The figure shows three views and two pictorial views of one solid part (mm, origin at its lowest corner). Answer the questions. A direction names the side the tool comes from. Coordinates: 2 decimals unless noted, no trailing zeros. Write each loop counter-clockwise with the first axis right and the second up, starting at its lowest first coordinate (ties: lowest second). Pieces come first, ordered by that corner, then holes. Notation, with made-up numbers: M 61,69.25 L 89,69.25 A28 cw 89,98.25 Z; hole C 70,26 d11. An arc over 180 degrees is marked long. Write item = value, one per line. Start each with the question number.
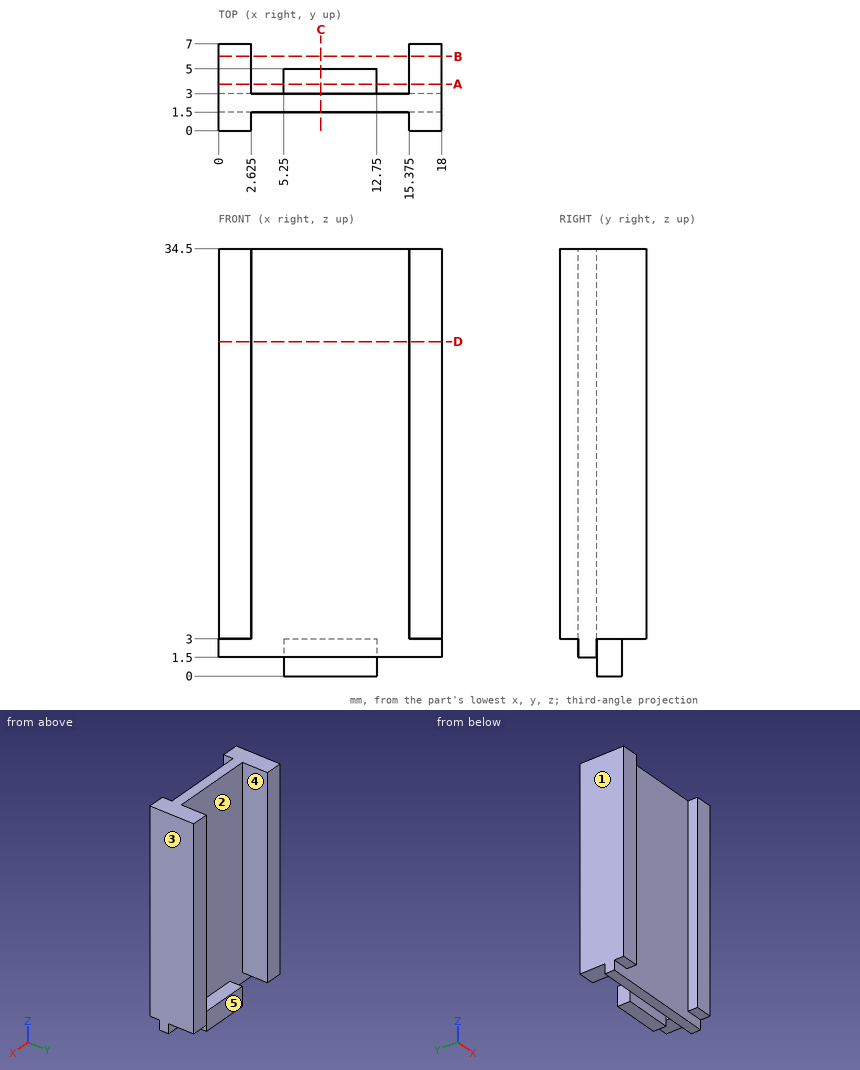
1. The part is cut by section D-D, the plane z = 27. Write down the section's boundary in (x, y) (3 decimals), and give its area (3 significant figures).
2. The part is cut by section B-B, the plane y = 6. Write down the section's boundary in (x, z) (3 decimals).
3. The part is cut by section A-A, the plane y = 3.75. Write down the section's boundary in (x, z) (3 decimals), and give its area (3 significant figures).
4. For the marked faces 4 and 5, determine the directions among +Z, -Z, +X, -X, +Y, -Y from which every point of the face is accessible in a straight line to the end or side of a thin tool.
5. Straight lines are drawn through the part: L1, parallel to X at y = 5, z = 3.5 (3 decimals); L2, parallel to Z at x = 9.75, y = 2.25; L3, parallel to Y at x = 9.25, z = 29. For each, find the intervals that lie inside material, in ascending order. Write a range as [from, to].
6. Each of these flat-tipped pins is pushed along its axis until it touches: pin 1 (6 mm diameter, centred on x = 15.5, z = 30, fed in from -Y); pin 2 (5 mm diameter, centred on x = 9, z = 23, fed in from +Y); pin 3 (1.6 mm diameter, centred on y = 4.5, z = 1.5, fed in from +X); pin 4 (2.5 mm diameter, centred on x = 8.5, z = 2, fed in from +Y). Where does it stop, or does it pass through?
7. For a pull along X with two mould halves and no side action, classify the marked faces 1, 2 and 3 as pulls with the +X half, pulls with the -X half, needs draft (parallel to the pull), parting line crosses it, or undercut.
8. The part is cut by section C-C, the plane x = 8.25. Write down the section's boundary in (y, z), and give its area (3 significant figures).
Solution:
q1.outline = M 0,0 L 2.625,0 L 2.625,1.5 L 15.375,1.5 L 15.375,0 L 18,0 L 18,7 L 15.375,7 L 15.375,3 L 2.625,3 L 2.625,7 L 0,7 Z
q1.area = 55.9 mm^2
q2.outline = M 0,3 L 2.625,3 L 2.625,34.5 L 0,34.5 Z; M 15.375,3 L 18,3 L 18,34.5 L 15.375,34.5 Z
q3.outline = M 0,3 L 2.625,3 L 2.625,34.5 L 0,34.5 Z; M 5.25,0 L 12.75,0 L 12.75,3 L 5.25,3 Z; M 15.375,3 L 18,3 L 18,34.5 L 15.375,34.5 Z
q3.area = 188 mm^2
q4.face_4 = +Z, -Z, +Y
q4.face_5 = +Z, -Z, +X, -X, +Y
q5.L1 = [0, 2.625], [15.375, 18]
q5.L2 = [1.5, 34.5]
q5.L3 = [1.5, 3]
q6.pin_1 = 0
q6.pin_2 = 3
q6.pin_3 = 12.75
q6.pin_4 = 5
q7.face_1 = pulls with the -X half
q7.face_2 = undercut
q7.face_3 = pulls with the +X half
q8.outline = M 1.5,1.5 L 3,1.5 L 3,0 L 5,0 L 5,3 L 3,3 L 3,34.5 L 1.5,34.5 Z
q8.area = 55.5 mm^2
